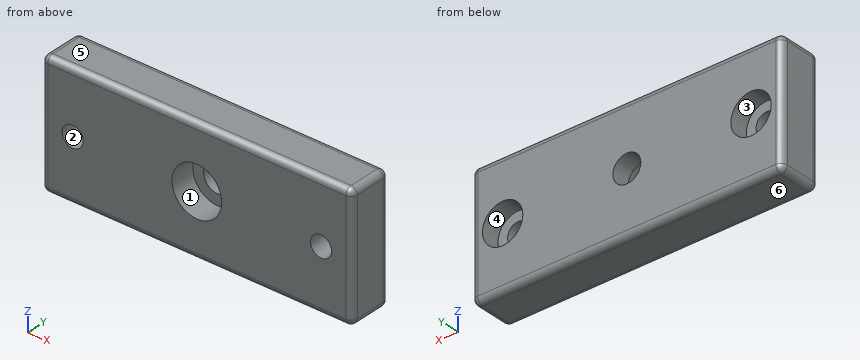
```python
from build123d import *

# Parameters (mm, degrees)
SKETCH1_W                      = 50
SKETCH1_H                      = 20
EXTRUDE1_DEPTH                 = 7
CBORE_FOR_M3_SHCS1_D           = 3.4
CBORE_FOR_M3_SHCS1_CBORE_D     = 6.5
CBORE_FOR_M3_SHCS1_CBORE_DEPTH = 3
FILLET1_R                      = 1
CBORE_FOR_M4_SHCS1_D           = 4.5
CBORE_FOR_M4_SHCS1_CBORE_D     = 8
CBORE_FOR_M4_SHCS1_CBORE_DEPTH = 4


with BuildPart() as part:
    # Sketch1 → Extrude1 (new body)
    with BuildSketch(Plane(origin=(0, 0, 0), x_dir=(1, 0, 0), z_dir=(0, 1, 0))):
        Rectangle(SKETCH1_W, SKETCH1_H)
    extrude(amount=EXTRUDE1_DEPTH)

    # CBORE for M3 SHCS1 (through all)
    with Locations(Plane(origin=(0, 7, 0), x_dir=(-1, 0, 0), z_dir=(0, 1, 0))):
        with Locations((20, 0), (-20, 0)):
            CounterBoreHole(CBORE_FOR_M3_SHCS1_D / 2, CBORE_FOR_M3_SHCS1_CBORE_D / 2, CBORE_FOR_M3_SHCS1_CBORE_DEPTH)

    # Fillet1
    fillet1_edges = [part.edges().sort_by_distance(p)[0] for p in [
        (25, 7, 0),
        (0, 7, -10),
        (-25, 7, 0),
        (0, 0, -10),
        (25, 0, 0),
        (0, 0, 10),
        (-25, 0, 0),
        (0, 7, 10),
        (-25, 3.5, -10),
        (25, 3.5, -10),
        (25, 3.5, 10),
        (-25, 3.5, 10),
    ]]
    fillet(fillet1_edges, radius=FILLET1_R)

    # CBORE for M4 SHCS1 (through all)
    with Locations(Plane(origin=(0, 0, 0), x_dir=(0, 0, -1), z_dir=(0, -1, 0))):
        with Locations((0, 0)):
            CounterBoreHole(CBORE_FOR_M4_SHCS1_D / 2, CBORE_FOR_M4_SHCS1_CBORE_D / 2, CBORE_FOR_M4_SHCS1_CBORE_DEPTH)


solid = part.part
```
Input: part model. Units: mm. Frame: model coordinates. Face numbers are marked on the shaded views. A direction names the side the tool comes from. Give positions to 0.01 mm unless a question says otherwise; leave off trailing zeros. Order: outer loops, then holes, each group sorted by start corner. A loop starts at its lowest first (then second) coordinate and runs counter-clockwise, first axis right, second up. Notation, with made-up numbers: (18, -39) - (39, -39) arc R19 cw to (39, -13) - close; hole circle Ø2 at (72, 52.5). An arc over 180 degrees is marked (long way). Use a Markdown table: item, result.
(1) Pin query (flat end, axial travel): pin 1 (3 mm diameter, centred on x = -20, z = -1.5, fed in from +Y); pin 2 (5 mm diameter, centred on x = 0, z = 0, fed in from -Y); pin 3 (9 mm diameter, centred on x = 1, z = 1.5, fed in from -Y). Return the tip coordinate at first contact, or that it passes through.
Computed values:
| item | result |
|---|---|
| pin 1 | stops at y = 4 |
| pin 2 | stops at y = 4 |
| pin 3 | stops at y = 0 |
(2) Access query for the marked faces 1, 2 and 3. Directions: +Z, -Z, +X, -X, +Y, -Y. A direction counts if a zero-diameter tool reaches every point of the face in a straight line with its end or side. Return the directions, or none.
Computed values:
| item | result |
|---|---|
| face 1 | -Y |
| face 2 | +Y, -Y |
| face 3 | +Y |
(3) Section query B-B (z = 0). State how many separate pieces and enclosed holes the cut face has, then the cut area to 3 significant figures.
Computed values:
| item | result |
|---|---|
| separate pieces | 4 |
| enclosed holes | 0 |
| area | 237 mm2 |
(4) Section query A-A (x = 20). Output: boundary loops of the cut face in (y, z), then the cut area to 3 significant figures.
Computed values:
| item | result |
|---|---|
| outline | (0, -9) arc R1 ccw to (1, -10) - (6, -10) arc R1 ccw to (7, -9) - (7, -3.25) - (4, -3.25) - (4, -1.7) - (0, -1.7) - close; (0, 1.7) - (4, 1.7) - (4, 3.25) - (7, 3.25) - (7, 9) arc R1 ccw to (6, 10) - (1, 10) arc R1 ccw to (0, 9) - close |
| area | 106 mm2 |
(5) Draft query along Z for the marked faces 4, 5 and 6. Return one class per face: released by +Z, released by -Z, zero draft, split by the parting line, or undercut.
Computed values:
| item | result |
|---|---|
| face 4 | undercut |
| face 5 | released by +Z |
| face 6 | released by -Z |
(6) Line query: line 1 (X direction, y = 5.5, z = -2.75); line 2 (Z direction, x = -20, y = 2.6); line 3 (Z direction, x = 20, y = 5.1). Output: solid intervals per line, ascending. Write a range as from..to.
Computed values:
| item | result |
|---|---|
| line 1 | x = -25..-21.73, -18.27..18.27, 21.73..25 |
| line 2 | z = -10..-1.7, 1.7..10 |
| line 3 | z = -10..-3.25, 3.25..10 |
(7) Section query D-D (x = 0). Output: boundary loops of the cut face in (y, z), then the cut area to 3 significant figures.
Computed values:
| item | result |
|---|---|
| outline | (0, -9) arc R1 ccw to (1, -10) - (6, -10) arc R1 ccw to (7, -9) - (7, -2.25) - (4, -2.25) - (4, -4) - (0, -4) - close; (0, 4) - (4, 4) - (4, 2.25) - (7, 2.25) - (7, 9) arc R1 ccw to (6, 10) - (1, 10) arc R1 ccw to (0, 9) - close |
| area | 93.6 mm2 |
(8) Section query C-C (y = 4.75). Output: boundary loops of the cut face in (x, z), then the cut area to 3 significant figures.
Computed values:
| item | result |
|---|---|
| outline | (-25, -9) arc R1 ccw to (-24, -10) - (24, -10) arc R1 ccw to (25, -9) - (25, 9) arc R1 ccw to (24, 10) - (-24, 10) arc R1 ccw to (-25, 9) - close; hole circle Ø6.5 at (-20, 0); hole circle Ø4.5 at (0, 0); hole circle Ø6.5 at (20, 0) |
| area | 917 mm2 |
